Can you work these out from the model? Positions are in its coordinate system, mm. Coordinates: 2 decimals unless noted, no trailing zeros. Order: outer loops, then holes, each group sorted by start corner. A loop starts at its lowest first (then second) coordinate and runs counter-clockwise, first axis right, second up. Notation, with made-up numbers: (55, 78.25) - (108, 78.25) arc R10 cw to (108, 82.25) - close; hole circle Ø4 at (-14, 39.5). An arc over 180 degrees is marked (long way). Return JSON: item names as keys, results as strings. Group by question number.
1) Imagine slicing it at B-B (y = -12). Write out the boundary of the cut face in (x, z).
2) If I drill on line 1 along Y through (x, z) = (15, 0.65); line 2 along X through (y, z) = (-12, 0.35); line 3 along Y through (x, z) = (-16, 0.55), over which ranges is the centre line in solid material (lowest first)?
3) Imagine slicing it at A-A (z = 0.15). Write out the boundary of the cut face in (x, y), and give its area (3 significant figures).
4) Imagine slicing it at C-C (x = -15). Write out the boundary of the cut face in (y, z), and give its area (3 significant figures).
5) For pin 1 Ø2.5 at (x, y) = (15, -12) entering from -Z; pin 2 Ø3 at (x, y) = (-10.5, 8.5) entering from -Z, each with a flat end and sliding along its axis, tell me the tip position at first contact or that it passes through.
Autodesk Inventor part; units mm, degrees
ref_plane "YZ Plane" through (0, 0, 0) normal (1, 0, 0) x (0, 1, 0)
ref_plane "XZ Plane" through (0, 0, 0) normal (0, 1, 0) x (-1, 0, 0)
ref_plane "XY Plane" through (0, 0, 0) normal (0, 0, 1) x (1, 0, 0)
sketch "草图1" plane through (0, 0, 0) normal (0, 0, 1) x (1, 0, 0)
  line L0 (18.5, -15.5) -> (-18.5, -15.5)
  line L1 (-18.5, -15.5) -> (-18.5, 15.5)
  line L2 (-18.5, 15.5) -> (18.5, 15.5)
  line L3 (18.5, 15.5) -> (18.5, -15.5)
  line L4 (18.5, -15.5) -> (-18.5, 15.5) construction
  line L5 (-18.5, -15.5) -> (18.5, 15.5) construction
  line L6 (0, 0) -> (-24.9379, 0) construction
  line L7 (0, 0) -> (0, 16.8364) construction
  point P0 (-15, 12)
  point P1 (-15, -12)
  point P2 (15, 12)
  point P3 (15, -12)
  dimension "d0" = 31
  dimension "d1" = 37
  dimension "d2" = 12
  dimension "d3" = 15
extrude "拉伸1" add sketch "草图1" along normal blind 1
hole "孔1" at (-15, 12, 0) at (-15, -12, 0) at (15, 12, 0) at (15, -12, 0) direction (0, 0, 1) diameter 4.2 end through all
properties part number "自制垫片"
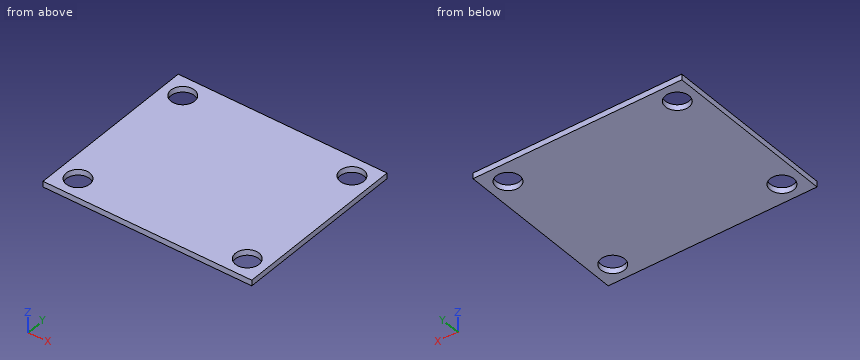
Calculated:
{
 "1": {"outline": "(-18.5, 0) - (-17.1, 0) - (-17.1, 1) - (-18.5, 1) - close; (-12.9, 0) - (12.9, 0) - (12.9, 1) - (-12.9, 1) - close; (17.1, 0) - (18.5, 0) - (18.5, 1) - (17.1, 1) - close"},
 "2": {"line 1": "-15.5 to -14.1, -9.9 to 9.9, 14.1 to 15.5", "line 2": "-18.5 to -17.1, -12.9 to 12.9, 17.1 to 18.5", "line 3": "-15.5 to -13.85, -10.15 to 10.15, 13.85 to 15.5"},
 "3": {"outline": "(-18.5, -15.5) - (18.5, -15.5) - (18.5, 15.5) - (-18.5, 15.5) - close; hole circle Ø4.2 at (-15, -12); hole circle Ø4.2 at (-15, 12); hole circle Ø4.2 at (15, -12); hole circle Ø4.2 at (15, 12)", "area": "1,090 mm2"},
 "4": {"outline": "(-15.5, 0) - (-14.1, 0) - (-14.1, 1) - (-15.5, 1) - close; (-9.9, 0) - (9.9, 0) - (9.9, 1) - (-9.9, 1) - close; (14.1, 0) - (15.5, 0) - (15.5, 1) - (14.1, 1) - close", "area": "22.6 mm2"},
 "5": {"pin 1": "through", "pin 2": "z = 0"}
}
